Autodesk Inventor part; units mm, degrees
ref_plane "YZ Plane" through (0, 0, 0) normal (1, 0, 0) x (0, 1, 0)
ref_plane "XZ Plane" through (0, 0, 0) normal (0, 1, 0) x (-1, 0, 0)
ref_plane "XY Plane" through (0, 0, 0) normal (0, 0, 1) x (1, 0, 0)
sketch "Sketch4" plane through (0, 0, 0) normal (0, 0, 1) x (1, 0, 0)
  line L0 (15.875, 9.525) -> (15.875, -9.525)
  line L1 (15.875, -9.525) -> (-15.875, -9.525)
  line L2 (-15.875, -9.525) -> (-15.875, 9.525)
  line L3 (-15.875, 9.525) -> (-11.1125, 9.525)
  line L4 (-11.1125, 9.525) -> (-11.1125, 15.875)
  line L5 (-11.1125, 15.875) -> (-4.7625, 15.875)
  line L6 (-4.7625, 15.875) -> (-4.7625, 9.525)
  line L7 (-4.7625, 9.525) -> (15.875, 9.525)
  line L8 (1.5875, 22.225) -> (-17.4625, 22.225)
  line L9 (-17.4625, 22.225) -> (-17.4625, 15.875)
  line L10 (-17.4625, 15.875) -> (-22.225, 15.875)
  line L11 (-22.225, 15.875) -> (-22.225, -15.875)
  line L12 (-22.225, -15.875) -> (22.225, -15.875)
  line L13 (22.225, -15.875) -> (22.225, 15.875)
  line L14 (22.225, 15.875) -> (1.5875, 15.875)
  line L15 (1.5875, 15.875) -> (1.5875, 22.225)
  circle A0 centre (-14.2875, 19.05) radius 1.27
  circle A1 centre (-1.5875, 19.05) radius 1.27
  circle A2 centre (-1.5875, 12.7) radius 1.27
  circle A3 centre (7.9375, 12.7) radius 1.27
  circle A4 centre (19.05, 12.7) radius 1.27
  circle A5 centre (19.05, 0) radius 1.27
  circle A6 centre (19.05, -12.7) radius 1.27
  circle A7 centre (-19.05, 0) radius 1.27
  circle A8 centre (-19.05, -12.7) radius 1.27
  circle A9 centre (-9.525, -12.7) radius 1.27
  circle A10 centre (0, -12.7) radius 1.27
  circle A11 centre (9.525, -12.7) radius 1.27
  circle A12 centre (-19.05, 12.7) radius 1.27
  point P0 (0, 0)
  dimension "d95" = 2.54
  dimension "d96" = 2.54
  dimension "d97" = 2.54
  dimension "d98" = 2.54
  dimension "d99" = 2.54
  dimension "d100" = 2.54
  dimension "d101" = 2.54
  dimension "d102" = 2.54
  dimension "d103" = 2.54
  dimension "d104" = 2.54
  dimension "d105" = 2.54
  dimension "d106" = 2.54
  dimension "d107" = 3.175
  dimension "d108" = 3.175
  dimension "d109" = 3.175
  dimension "d110" = 3.175
  dimension "d111" = 3.175
  dimension "d112" = 3.175
  dimension "d113" = 9.525
  dimension "d114" = 9.525
  dimension "d115" = 9.525
  dimension "d116" = 9.525
  dimension "d117" = 2.54
  dimension "d118" = 3.175
  dimension "d119" = 3.175
extrude "Extrusion4" add sketch "Sketch4" along normal blind 3.175 contours L0 L1 L2 L3 L4 L5 L6 L7 | L15 L14 L13 L12 L11 L10 L9 L8
chamfer "Chamfer4" distance 1.27 angle 45 13 edges at (-15.5575, 19.05, 3.175) (-2.8575, 19.05, 3.175) (-2.8575, 12.7, 3.175) (6.6675, 12.7, 3.175) (17.78, 12.7, 3.175) (17.78, 0, 3.175) (17.78, -12.7, 3.175) (8.255, -12.7, 3.175) (-1.27, -12.7, 3.175) (-10.795, -12.7, 3.175) (-20.32, -12.7, 3.175) (-20.32, 0, 3.175) (-20.32, 12.7, 3.175)
fillet "Fillet3" radius 3.175 8 edges at (-17.4625, 22.225, 1.5875) (1.5875, 22.225, 1.5875) (1.5875, 15.875, 1.5875) (-17.4625, 15.875, 1.5875) (-22.225, 15.875, 1.5875) (22.225, 15.875, 1.5875) (22.225, -15.875, 1.5875) (-22.225, -15.875, 1.5875)
equation "\"d115\" = d114"
equation "\"d116\" = d114"
properties part number "foreElectronicsSealingWallFrontCap" material "ABS Plastic"
Could you check a few things on this model? Use its own coordinates, in mm. A direction names the side the tool comes from. Coordinates: 2 decimals unless noted, no trailing zeros.
Q1. Please list where these lines run through material, in increasing order: L1, parallel to Y at x = 10.5, z = 2.85 (3 decimals); L2, parallel to X at y = 0.5, z = 1.4 (3 decimals); L3, parallel to Y at x = 15.5, z = 0.7 (3 decimals).
Q2. Will these pins go through, and if not, where does the flat tip stop? pin 1 (4 mm diameter, centred on x = -19.05, y = 0, fed in from +Z) (3 decimals); pin 2 (3 mm diameter, centred on x = -14.29, y = 19.05, fed in from +Z).
Q3. Which directions (+Z, -Z, +X, -X, +Y, -Y) give clear straight access to the entire face, cutting with the end or side of a thin tool? Please do faces 1 (the flat face through (0, -1, 3.175)), 2 (the flat face through (12, 15.875, 2)).
Q4. Suppose I cut it at A-A on z = 1.35. Give the number of separate pieces and of enclosed holes in the cut face, and give its area (3 significant figures).
Q5. Thinking about a two-plate mould opening in Y: for faces 3 (the flat face through (0, -15.875, 2)), 4 (the cylindrical face through (18.04, 13.47, 0.94)), 5 (the flat face through (0, 3, 0)), 6 (the cylindrical face through (21.32, 14.92, 1.61)), which applies, released by +Y, released by -Y, zero draft, split by the parting line, or undercut?
Answer:
1. L1: y = -15.875 to -14.689, -10.711 to 15.875
1. L2: x = -22.225 to -20.217, -17.883 to 17.883, 20.217 to 22.225
1. L3: y = -15.875 to 15.875
2. pin 1: stops at z = 2.635
2. pin 2: stops at z = 2.14
3. face 1: +Z, +X, -X, +Y, -Y
3. face 2: +Z, -Z, +X, +Y
4. separate pieces: 1
4. enclosed holes: 13
4. area: 1,460 mm2
5. face 3: released by -Y
5. face 4: undercut
5. face 5: zero draft
5. face 6: released by +Y
